Input: part model. Units: mm. Frame: model coordinates. A direction names the side the tool comes from. Round coordinates to 2 decimals unless told otherwise and drop trailing zeros. Answer as a JSON object with one key per item and string values. Group by question number.
Item 1: Material intervals for line 1 (X direction, y = -4.9, z = 0); line 2 (Z direction, x = -10.5, y = -7); line 3 (Z direction, x = -18.5, y = 0.5), sorted ascending. Write a range as [from, to].
Item 2: Pin query (flat end, axial travel): pin 1 (1.5 mm diameter, centred on x = 20.5, y = -6, fed in from +Z); pin 2 (10 mm diameter, centred on x = -12, z = -15.5, fed in from +Y); pin 3 (5 mm diameter, centred on y = -1.5, z = -12, fed in from +X); pin 4 (10 mm diameter, centred on x = -17, z = 0, fed in from -Y). Return the tip coordinate at first contact, or that it passes through.
Item 3: Set-up query: faces 1 (the cylindrical face through (-17.572, -4.22, 19.163)), 2 (the flat face through (11.7, 0, -18.3)). Return all of +Z, -Z, +X, -X, +Y, -Y with unobstructed straight access to the full face (end or side cutting, diameter ignored); none if empty.
Item 4: Draft query along Y for faces 3 (the cylindrical face through (-23.726, -7.746, 3.115)), 4 (the flat face through (17.2, -8, -17.2)), 5 (the cylindrical face through (-23.726, -6.219, 3.115)), 6 (the cylindrical face through (9.09, -2.29, -21.93)). Return one class per face: released by +Y, released by -Y, zero draft, split by the parting line, or undercut.
from build123d import *

# Parameters (mm, degrees)
SKETCH_1_R               = 26
EXTRUDE_1_DEPTH          = 2
SKETCH_5_R               = 21.5
CUT_EXTRUDE_1_DEPTH      = 39.105117767
CUT_EXTRUDE_START        = -0.6
SKETCH_7_R               = 26
CUT_EXTRUDE_2_DEPTH      = 0.6
CHAMFER_1_SIZE           = 1.732
CHAMFER_1_SIZE2          = 0.999970666
CHAMFER_2_SIZE           = 1.2
CUT_REVOLVE_1_ANGLE      = 45
PATTERN_CIRCULAR_1_COUNT = 4
SKETCH_9_R               = 22.78
SKETCH_9_R_2             = 22.32
EXTRUDE_2_DEPTH          = 0.5


with BuildPart() as part:
    # 草图1 → 凸台-拉伸1 (new body)
    with BuildSketch(Plane(origin=(0, 0, 0), x_dir=(1, 0, 0), z_dir=(0, 1, 0))):
        with Locations(Location((0, 0, 0), (0, 0, 270))):
            Circle(SKETCH_1_R)
    extrude(amount=EXTRUDE_1_DEPTH)

    # 草图4 → 旋转1 (revolve)
    with BuildSketch(Plane(origin=(0, 0, 0), x_dir=(0.8660254037844574, 0, 0.4999999999999675), z_dir=(-0.4999999999999675, 0, 0.8660254037844574)), mode=Mode.PRIVATE) as revolve_1_sk:
        with BuildLine():
            Line((23.93, -8), (23.93, -7.5))
            Line((23.93, -7.5), (23.505, -7.075))
            Line((23.505, -7.075), (23.93, -6.65))
            Line((23.93, -6.65), (23.93, -5.8))
            Line((23.93, -5.8), (23.74, -5.61))
            Line((23.74, -5.61), (23.74, -4.59))
            Line((23.74, -4.59), (23.93, -4.4))
            Line((23.93, -4.4), (23.93, -3))
            Line((23.93, -3), (23.74, -2.81))
            Line((23.74, -2.81), (23.74, -1.79))
            Line((23.74, -1.79), (23.93, -1.6))
            Line((23.93, -1.6), (23.93, -1.4))
            ThreePointArc((23.93, -1.4), (23.519949494, -0.410050506), (22.53, 0))
            Line((22.53, 0), (26, 0))
            Line((26, 0), (26, -8))
            Line((26, -8), (23.93, -8))
        make_face()
    revolve(revolve_1_sk.sketch.rotate(Axis((0, 0, 0), (0, 1, 0)), 120), axis=Axis((0, 0, 0), (0, 1, 0)))

    # 草图5 → 切除-拉伸1 (cut, through all)
    with BuildSketch(Plane(origin=(0, 2, 0), x_dir=(1, 0, 0), z_dir=(0, 1, 0))):
        with Locations(Location((0, 0, 0), (0, 0, 270))):
            Circle(SKETCH_5_R)
    extrude(amount=-CUT_EXTRUDE_1_DEPTH, mode=Mode.SUBTRACT)

    # 草图7 → 切除-拉伸2 (cut)
    with BuildSketch(Plane(origin=(0, 2, 0), x_dir=(1, 0, 0), z_dir=(0, 1, 0)).offset(CUT_EXTRUDE_START)):
        with Locations(Location((0, 0, 0), (0, 0, 90))):
            Circle(SKETCH_7_R)
    extrude(amount=CUT_EXTRUDE_2_DEPTH, mode=Mode.SUBTRACT)

    # 倒角1
    chamfer_1_edges = [part.edges().sort_by_distance(p)[0] for p in [
        (0, 1.4, -26),
    ]]
    chamfer_1_side = [part.faces().sort_by_distance(p)[0] for p in [
        (26, -3.3, 0),
    ]]
    chamfer(chamfer_1_edges, length=CHAMFER_1_SIZE, length2=CHAMFER_1_SIZE2, reference=chamfer_1_side[0])

    # 倒角2
    chamfer_2_edges = [part.edges().sort_by_distance(p)[0] for p in [
        (0, 1.4, -21.5),
    ]]
    chamfer(chamfer_2_edges, length=CHAMFER_2_SIZE)

    # 草图8 → 切除-旋转1 (revolve, cut)
    with BuildSketch(Plane.XY):
        Polygon((26, -8), (26, -7), (25, -8), align=None)
    cut_revolve_1 = revolve(axis=Axis((0, 0, 0), (0, 1, 0)), revolution_arc=CUT_REVOLVE_1_ANGLE, mode=Mode.SUBTRACT)

    # 阵列(圆周)1: 切除-旋转1 ×4 about axis
    pattern_circular_1_axis = Axis((0, 0, 0), (0, 1, 0))
    for i in range(1, PATTERN_CIRCULAR_1_COUNT):
        add(cut_revolve_1.rotate(pattern_circular_1_axis, i * 360 / PATTERN_CIRCULAR_1_COUNT), mode=Mode.SUBTRACT)

    # 草图9 → 凸台-拉伸2 (add)
    with BuildSketch(Plane.XZ):
        with Locations(Location((0, 0, 0), (0, 0, 270))):
            Circle(SKETCH_9_R)
        with Locations(Location((0, 0, 0), (0, 0, 270))):
            Circle(SKETCH_9_R_2, mode=Mode.SUBTRACT)
    extrude(amount=EXTRUDE_2_DEPTH)


solid = part.part
Solved:
{
 "1": {"line 1": "[-26, -23.74], [23.74, 26]", "line 2": "[-23.79, -21.11], [21.11, 23.79]", "line 3": "[-17.58, -11.53], [11.53, 17.58]"},
 "2": {"pin 1": "z = 16.91", "pin 2": "y = 1.4", "pin 3": "x = 24.2", "pin 4": "y = 0"},
 "3": {"face 1": "+Y, -Y", "face 2": "-Y"},
 "4": {"face 3": "zero draft", "face 4": "released by -Y", "face 5": "undercut", "face 6": "undercut"}
}
